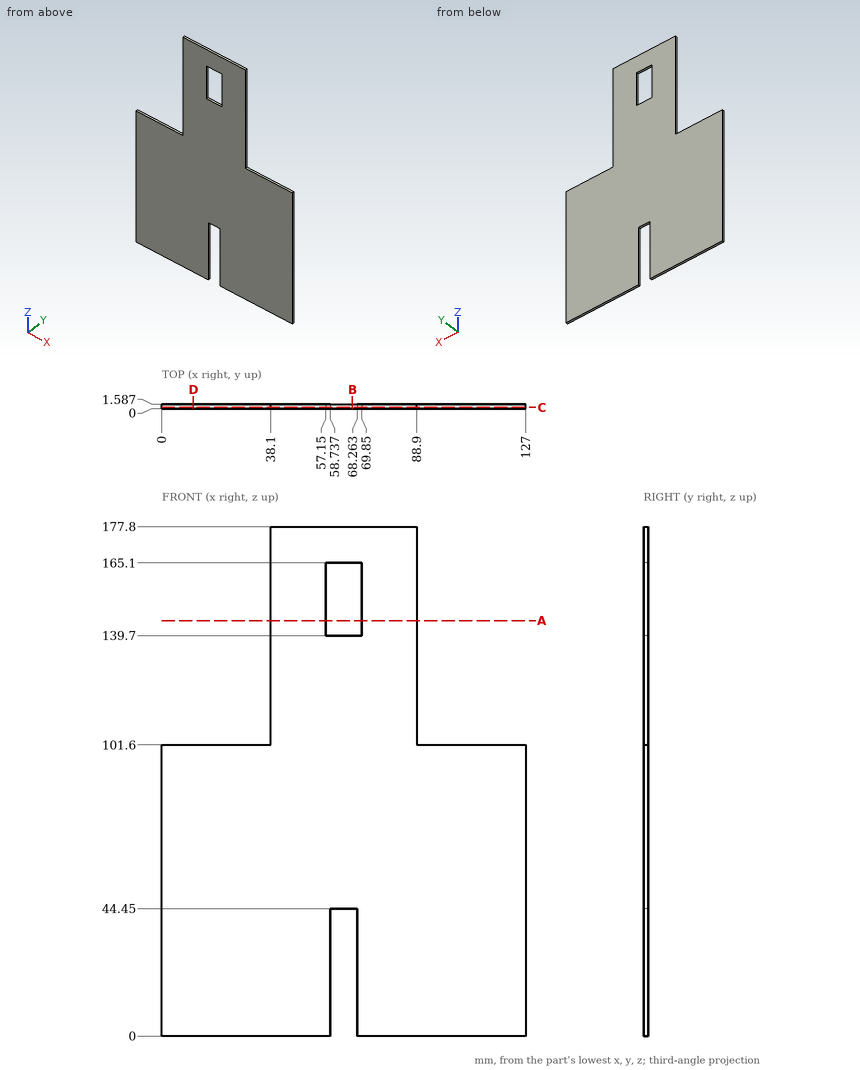
Geometry: see drawing. Coordinates: mm, zero at the bounding-box minimum. Round coordinates to 2 decimals unless told otherwise and drop trailing zeros. Order: outer loops, then holes, each group sorted by start corner. A loop starts at its lowest first (then second) coordinate and runs counter-clockwise, first axis right, second up. Notation, with made-up numbers: (64.5, 71) -> (99.5, 71) arc R13 ccw to (99.5, 85) -> close; hole circle Ø2 at (-22, 18.5). An arc over 180 degrees is marked (long way). Use CSV: the item, a comma, the result in double quotes.
(1) Section B-B on x = 66.5. Return the cut outline in (y, z).
Report:
outline,"(0, 44.45) -> (1.59, 44.45) -> (1.59, 139.7) -> (0, 139.7) -> close; (0, 165.1) -> (1.59, 165.1) -> (1.59, 177.8) -> (0, 177.8) -> close"
(2) Section D-D on x = 11. Return the cut outline in (y, z), and give its area (3 significant figures).
Report:
outline,"(0, 0) -> (1.59, 0) -> (1.59, 101.6) -> (0, 101.6) -> close"
area,"161 mm^2"
(3) First-contact query: pin 1 Ø0.5 at (x, y) = (114, 1) entering from +Z; pin 2 Ø0.5 at (y, z) = (1, 121.5) entering from -X; pin 3 Ø0.5 at (x, y) = (64, 1) entering from -Z. Flat tips, straight axial feed; report the tip coordinate or a pass-through.
Report:
pin 1,"z = 101.6"
pin 2,"x = 38.1"
pin 3,"z = 44.45"
(4) Section C-C on y = 0.4. Return the cut outline in (x, z).
Report:
outline,"(0, 0) -> (58.74, 0) -> (58.74, 44.45) -> (68.26, 44.45) -> (68.26, 0) -> (127, 0) -> (127, 101.6) -> (88.9, 101.6) -> (88.9, 177.8) -> (38.1, 177.8) -> (38.1, 101.6) -> (0, 101.6) -> close; hole (57.15, 139.7) -> (69.85, 139.7) -> (69.85, 165.1) -> (57.15, 165.1) -> close"
(5) Ray query, L1, parallel to X at y = 1.4, z = 12.5; L2, parallel to X at y = 1.2, z = 119.5; L3, parallel to Z at x = 38, y = 1. Return the intervals inside material, ascending.
Report:
L1,"0 to 58.74, 68.26 to 127"
L2,"38.1 to 88.9"
L3,"0 to 101.6"
(6) Section A-A on z = 145. Return the cut outline in (x, y).
Report:
outline,"(38.1, 0) -> (57.15, 0) -> (57.15, 1.59) -> (38.1, 1.59) -> close; (69.85, 0) -> (88.9, 0) -> (88.9, 1.59) -> (69.85, 1.59) -> close"
